Source: CAD feature listing. Evaluate the final solid. Frame: model axes, mm. Face numbers are marked on the shaded views. A direction names the side the tool comes from. Give positions to 0.01 mm unless a question says otherwise; leave off trailing zeros. Order: outer loops, then holes, each group sorted by start corner. A loop starts at its lowest first (then second) coordinate and runs counter-clockwise, first axis right, second up.
from build123d import *

# Parameters (mm, degrees)
F0_R     = 10
F1_DEPTH = 10
F3_DEPTH = 10


with BuildPart() as f1:
    # F0 (on Front) → F1 (new body)
    with BuildSketch(Plane.XZ):
        with BuildLine():
            Line((0, 20), (0, 0))
            Line((0, 0), (20, 0))
            Line((20, 0), (60, 0))
            Line((60, 0), (60, 10))
            ThreePointArc((60, 10), (57.071068, 17.071068), (50, 20))
            Line((50, 20), (40, 20))
            ThreePointArc((40, 20), (20, 40), (0, 20))
        make_face()
        with Locations((20, 20)):
            Circle(F0_R, mode=Mode.SUBTRACT)
    extrude(amount=-F1_DEPTH)

    # F2 (on face) → F3 (join)
    with BuildSketch(Plane(origin=(0, 10, 0), x_dir=(-1, 0, 0), z_dir=(0, 1, 0))):
        Polygon((-60, 0), (0, 0), (0, 10), (-20, 10), (-60, 10), align=None)
    extrude(amount=F3_DEPTH)


solid = f1.part
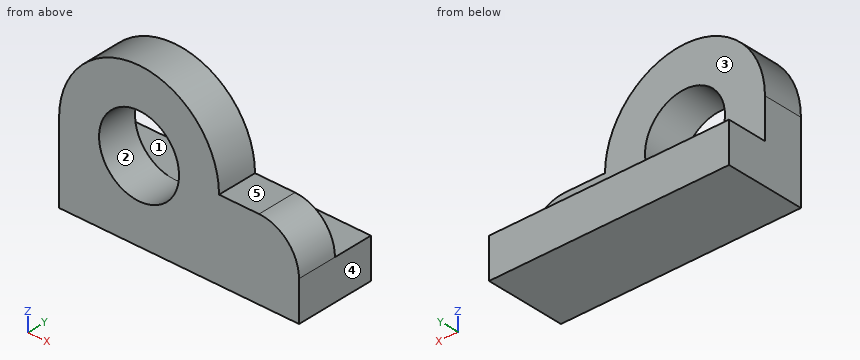
(1) Line query: line 1 along Y through (x, z) = (57.5, 14); line 2 along Z through (x, y) = (20, 4.75). Output: solid intervals per line, ascending.
(2) Section B-B, the plane x = 12. Return loops of the section in (y, z), plus the area to 3 significant figures.
(3) Access query for the marked faces 4 and 5. Directions: +Z, -Z, +X, -X, +Y, -Y. A direction counts if a zero-diameter tool reaches every point of the face in a straight line with its end or side. Return the directions, or none.
(4) Pin query (flat end, axial travel): pin 1 Ø18 at (x, z) = (20, 20) entering from +Y; pin 2 Ø1.5 at (y, z) = (6, 30) entering from -X; pin 3 Ø3 at (x, y) = (45.5, 4.5) entering from +Z. Return the tip coordinate at first contact, or that it passes through.
(5) Section C-C, the plane x = 4. Return loops of the section in (y, z).
(6) Draft query along Z for the marked faces 1, 2 and 3. Return one class per face: +Z half, -Z half, draft (parallel to the pull), parting line (faces both ways), or undercut.
(7) Section A-A, the plane y = 9. Return loops of the section in (x, z), plus the area to 3 significant figures.
(8) Section D-D, the plane z = 36. Return loops of the section in (x, y), plus the area to 3 significant figures.
Checks:
1. line 1: y = 0 to 10
1. line 2: z = 0 to 10, 30 to 40
2. outline: (0, 0) - (20, 0) - (20, 10) - (10, 10) - (10, 14) - (0, 14) - close; (0, 26) - (10, 26) - (10, 38.33) - (0, 38.33) - close
2. area: 363 mm2
3. face 4: +Z, -Z, +X, +Y, -Y
3. face 5: +Z, +X, +Y, -Y
4. pin 1: passes through
4. pin 2: stops at x = 2.27
4. pin 3: stops at z = 20
5. outline: (0, 0) - (20, 0) - (20, 10) - (10, 10) - (10, 32) - (0, 32) - close
6. face 1: +Z half
6. face 2: undercut
6. face 3: draft
7. outline: (0, 0) - (60, 0) - (60, 10) arc R10 ccw to (50, 20) - (40, 20) arc R20 ccw to (0, 20) - close; hole circle Ø20 at (20, 20)
7. area: 1,490 mm2
8. outline: (8, 0) - (32, 0) - (32, 10) - (8, 10) - close
8. area: 240 mm2
